from build123d import *

# Parameters (mm, degrees)
SCHIZZO1_R                   = 2.5
SCHIZZO1_R_2                 = 2
ESTRUSIONE_ESTRUSIONE1_DEPTH = 10
TAGLIO_ESTRUSIONE1_DEPTH     = 76.013178039
SCHIZZO3_R                   = 2
TAGLIO_ESTRUSIONE2_DEPTH     = 76.013178039


with BuildPart() as part:
    # Schizzo1 → Estrusione-Estrusione1 (new body)
    with BuildSketch(Plane.XY):
        with BuildLine():
            Line((15, -50), (-35, -50))
            Line((-35, -50), (-35, -31.964890017))
            Line((-35, -31.964890017), (-55.017968697, -15.891116751))
            Line((-55.017968697, -15.891116751), (-55.017968697, -2.739847716))
            Line((-55.017968697, -2.739847716), (-23.966361252, 11.142047377))
            Line((-23.966361252, 11.142047377), (-23.966361252, 14.909560068))
            ThreePointArc((-23.966361252, 14.909560068), (-22.501895158, 18.445093974), (-18.966361252, 19.909560068))
            Line((-18.966361252, 19.909560068), (9.612052016, 19.909560068))
            ThreePointArc((9.612052016, 19.909560068), (21.117133083, 14.534169651), (24.376307149, 2.260641352))
            Line((24.376307149, 2.260641352), (15, -31.964890017))
            Line((15, -31.964890017), (15, -50))
        make_face()
        Circle(SCHIZZO1_R, mode=Mode.SUBTRACT)
        with Locations((-20, -45)):
            Circle(SCHIZZO1_R_2, mode=Mode.SUBTRACT)
        with Locations((0, -45)):
            Circle(SCHIZZO1_R_2, mode=Mode.SUBTRACT)
        with Locations((-49.725907234, -5.689936133)):
            Circle(SCHIZZO1_R_2, mode=Mode.SUBTRACT)
        with Locations((-49.850768961, -13.68896167)):
            Circle(SCHIZZO1_R_2, mode=Mode.SUBTRACT)
        with Locations((-18.966361252, 14.909560068)):
            Circle(SCHIZZO1_R_2, mode=Mode.SUBTRACT)
    extrude(amount=ESTRUSIONE_ESTRUSIONE1_DEPTH)

    # Schizzo2 → Taglio-Estrusione1 (cut, through all)
    with BuildSketch(Plane.XY.offset(10)):
        with BuildLine():
            Line((-27.856099407, -12.90456221), (-2.268412004, -1.050860115))
            ThreePointArc((-2.268412004, -1.050860115), (-1.050860115, 2.268412004), (2.268412004, 1.050860115))
            Line((2.268412004, 1.050860115), (9.073648015, 4.203440459))
            Line((9.073648015, 4.203440459), (4.870207556, 13.277088475))
            Line((4.870207556, 13.277088475), (-32.059539866, -3.830914194))
            Line((-32.059539866, -3.830914194), (-27.856099407, -12.90456221))
        make_face()
        with BuildLine():
            ThreePointArc((2.5, 0), (0.538038098, -2.441416598), (-2.268412004, -1.050860115))
            Line((-2.268412004, -1.050860115), (-27.856099407, -12.90456221))
            Line((-27.856099407, -12.90456221), (-23.652658948, -21.978210225))
            Line((-23.652658948, -21.978210225), (13.277088475, -4.870207556))
            Line((13.277088475, -4.870207556), (9.073648015, 4.203440459))
            Line((9.073648015, 4.203440459), (2.268412004, 1.050860115))
            ThreePointArc((2.268412004, 1.050860115), (2.441416598, 0.538038098), (2.5, 0))
        make_face()
    extrude(amount=-TAGLIO_ESTRUSIONE1_DEPTH, mode=Mode.SUBTRACT)

    # Schizzo3 → Taglio-Estrusione2 (cut, through all)
    with BuildSketch(Plane.XY.offset(10)):
        with Locations((10.601386992, 10.421640651)):
            Circle(SCHIZZO3_R)
        with Locations((14.804827451, 1.347992635)):
            Circle(SCHIZZO3_R)
        with Locations((-29.383838384, -19.122762401)):
            Circle(SCHIZZO3_R)
        with Locations((-33.587278843, -10.049114386)):
            Circle(SCHIZZO3_R)
    extrude(amount=-TAGLIO_ESTRUSIONE2_DEPTH, mode=Mode.SUBTRACT)


solid = part.part
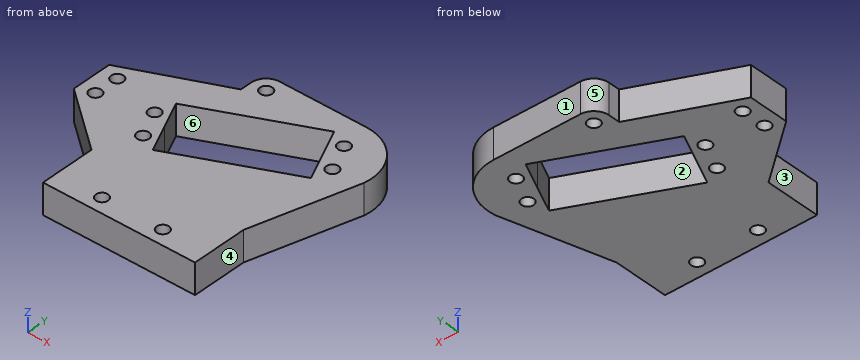
Check sheet for the modelled part. Datum: model origin and axes. Units: mm. Face numbers are marked on the shaded views. A direction names the side the tool comes from. Round coordinates to 2 decimals unless told otherwise and drop trailing zeros. Loops run counter-clockwise (first coordinate to the right, second up) from the corner with the lowest first, then second, coordinate; pieces in that order, holes last. Notation, with made-up numbers: M 75,-18.5 L 99,-18.5 A28 cw 99,19.5 Z; hole C 89.5,-37 d8. An arc over 180 degrees is marked long. One line per question, with ' | ' between items. Start each with the question number.
Item 1: Section check D-D (z = 4). State how many separate pieces and enclosed holes the cut face has, and give its area (3 significant figures).
Item 2: Scan lines: probe 1 along X at (y, z) = (-12.5, 6.75); probe 2 along Y at (x, z) = (-30, 1); probe 3 along Y at (x, z) = (13, 7.25). Record each from-to range of solid material in increasing order.
Item 3: Gauge pin test, flat ends, axial feed: pin 1 Ø3.5 at (x, y) = (-29.38, -19.12) entering from +Z; pin 2 Ø1.5 at (x, z) = (-20.5, 8) entering from +Y; pin 3 Ø5 at (x, z) = (-43, 8) entering from +Y; pin 4 Ø3 at (y, z) = (13, 6) entering from -X. Record the tip position at first contact, or that the pin passes through.
Item 4: Section check B-B (y = -45). Record the boundary of the cut face in (x, z), and give its area (3 significant figures).
Item 5: Set-up check for the marked faces 4, 5 and 6: record each of +Z, -Z, +X, -X, +Y, -Y from which the full face is reachable in a straight line by a thin tool's end or side.
Item 6: Release check for a two-part mould opening along X. For the marked faces 1, 2 and 3 record: released by +X, released by -X, zero draft, split by the parting line, or undercut.
Item 7: Section check A-A (x = 0). Record the boundary of the cut face in (y, z), and give its area (3 significant figures).
Item 8: Section check C-C (x = -33). Record the boundary of the cut face in (y, z), and give its area (3 significant figures).
Worked out:
1) separate pieces: 1 | enclosed holes: 10 | area: 3,230 mm^2
2) probe 1: -55.02 to -51.46, -48.24 to -28.04, -3.19 to 20.33 | probe 2: -50 to -21.03, -17.22 to -8.28, -2.88 to 8.44 | probe 3: -50 to -5, -4.27 to 0.49, 2.21 to 19.52
3) pin 1: through | pin 2: y = 19.85 | pin 3: y = 3.75 | pin 4: x = -23.97
4) outline: M -35,0 L -22,0 L -22,10 L -35,10 Z; M -18,0 L -2,0 L -2,10 L -18,10 Z; M 2,0 L 15,0 L 15,10 L 2,10 Z | area: 420 mm^2
5) face 4: +Z, -Z, +X, -Y | face 5: +Z, -Z, -X, +Y | face 6: +Z, -Z
6) face 1: zero draft | face 2: undercut | face 3: released by -X
7) outline: M -50,0 L -47,0 L -47,10 L -50,10 Z; M -43,0 L -11.02,0 L -11.02,10 L -43,10 Z; M 11.02,0 L 19.91,0 L 19.91,10 L 11.02,10 Z | area: 439 mm^2
8) outline: M -50,0 L -11.96,0 L -11.96,10 L -50,10 Z; M -8.14,0 L 7.1,0 L 7.1,10 L -8.14,10 Z | area: 533 mm^2
